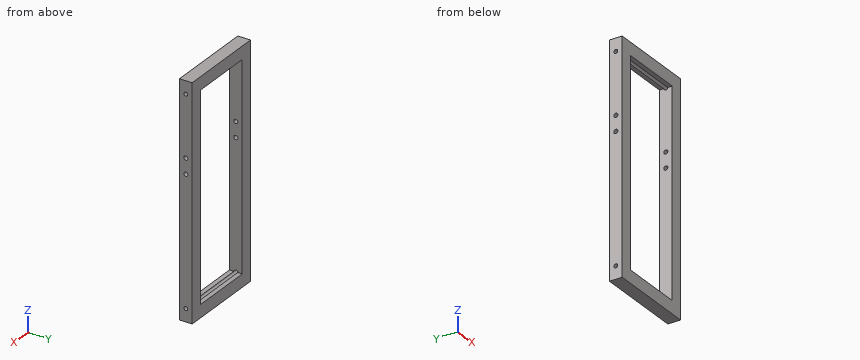
from build123d import *

# Parameters (mm, degrees)
CROQUIS1_W                   = 70
CROQUIS1_H                   = 180
CROQUIS1_W_2                 = 50
CROQUIS1_H_2                 = 160
SALIENTE_EXTRUIR1_DEPTH      = 5
CROQUIS2_R                   = 1.5
CORTAR_EXTRUIR1_DEPTH        = 60
TALADRO_DE_MARGEN_PARA_M31_D = 3.2


with BuildPart() as part:
    # Croquis1 → Saliente-Extruir1 (new, symmetric)
    with BuildSketch(Plane(origin=(0, 0, 0), x_dir=(1, 0, 0), z_dir=(0, 1, 0))):
        Rectangle(CROQUIS1_W, CROQUIS1_H)
        Rectangle(CROQUIS1_W_2, CROQUIS1_H_2, mode=Mode.SUBTRACT)
    extrude(amount=SALIENTE_EXTRUIR1_DEPTH, both=True)

    # Croquis2 → Cortar-Extruir1 (cut, symmetric)
    with BuildSketch(Plane(origin=(0, 0, 0), x_dir=(0, 0, -1), z_dir=(1, 0, 0))):
        with Locations((-80, 0)):
            Circle(CROQUIS2_R)
        with Locations((80, 0)):
            Circle(CROQUIS2_R)
    extrude(amount=CORTAR_EXTRUIR1_DEPTH, both=True, mode=Mode.SUBTRACT)

    # Taladro de margen para M31 (through all)
    with Locations(Plane(origin=(-35, -0.010928271, 32.287523851), x_dir=(0, 0, -1), z_dir=(-1, 0, 0))):
        with Locations((0, 0), (12.001709214, -0.007929279)):
            Hole(TALADRO_DE_MARGEN_PARA_M31_D / 2)


solid = part.part
For this review, take the finished solid that the model builds, in its own axes (mm). Coordinates: 2 decimals unless noted, no trailing zeros. Order: outer loops, then holes, each group sorted by start corner. A loop starts at its lowest first (then second) coordinate and runs counter-clockwise, first axis right, second up. Notation, with made-up numbers: (57.5, 61.5) - (73.5, 61.5) arc R12 ccw to (73.5, 74.5) - close; hole circle Ø8 at (77.25, -7.75). An arc over 180 degrees is marked (long way). Use one line per item in the form item = value.
Q1. Consider section B-B (z = 0). Give the boundary of the cut face in (x, y), then the cut area to 3 significant figures.
Checked values:
outline = (-35, -5) - (-25, -5) - (-25, 5) - (-35, 5) - close; (25, -5) - (35, -5) - (35, 5) - (25, 5) - close
area = 200 mm2
Q2. Consider section A-A (x = -0.5). Give the boundary of the cut face in (y, z).
Checked values:
outline = (-5, -90) - (5, -90) - (5, -80) - (1.5, -80) arc R1.5 cw to (-1.5, -80) - (-5, -80) - close; (-5, 80) - (-1.5, 80) arc R1.5 cw to (1.5, 80) - (5, 80) - (5, 90) - (-5, 90) - close
Q3. For probe 1 along Z at (x, y) = (-19.5, -2.5); probe 2 along X at (y, z) = (0.5, 14.5); probe 3 along Z at (x, y) = (12, 0.25), list the stretches that pass through material, from the lowest coordinate up. Write a range as from..to.
Checked values:
probe_1 = -90..-80, 80..90
probe_2 = -35..-25, 25..35
probe_3 = -90..-81.48, 81.48..90
Q4. For P1, Ø4, axis at y = 0, z = 20.29, coming from the +X side, flat-tipped, find the tip position at first contact; note if it passes through.
Checked values:
P1 = 35
Q5. Consider section C-C (x = -29). Give the boundary of the cut face in (y, z).
Checked values:
outline = (-5, -90) - (5, -90) - (5, 90) - (-5, 90) - close; hole circle Ø3.2 at (-0.01, 32.29); hole circle Ø3.2 at (0, 20.29); hole circle Ø3 at (0, -80); hole circle Ø3 at (0, 80)
